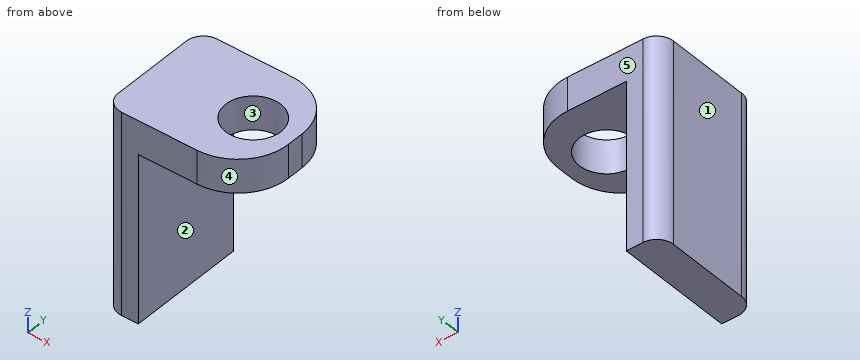
Autodesk Inventor part; units mm, degrees
ref_plane "YZ Plane" through (0, 0, 0) normal (1, 0, 0) x (0, 1, 0)
ref_plane "XZ Plane" through (0, 0, 0) normal (0, 1, 0) x (-1, 0, 0)
ref_plane "XY Plane" through (0, 0, 0) normal (0, 0, 1) x (1, 0, 0)
sketch "スケッチ1" plane through (0, 0, 0) normal (0, 0, 1) x (1, 0, 0)
  circle A0 centre (0, 0) radius 1.635
  line L0 (-6, -3.5) -> (2.5, -3.5)
  line L1 (2.5, -3.5) -> (2.5, 3.5)
  line L2 (2.5, 3.5) -> (-6, 3.5)
  line L3 (-6, 3.5) -> (-6, -3.5)
  line L4 (-6, -3.5) -> (2.5, 3.5) construction
  line L5 (2.5, -3.5) -> (-6, 3.5) construction
  line L6 (-6, 0) -> (2.5, 0) construction
  line L7 (-4, 3.5) -> (-4, -3.5)
  point P0 (-1.75, 0)
  dimension "d0" = 3.27
  dimension "d1" = 7
  dimension "d2" = 2.5
  dimension "d3" = 6
  dimension "d6" = 2
extrude "押し出し1" add sketch "スケッチ1" along normal blind 2
extrude "押し出し2" add sketch "スケッチ1" against normal blind 10 contours L3 L2 L7 L0
fillet "フィレット1" radius 3 2 edges at (2.5, 3.5, 1) (2.5, -3.5, 1)
fillet "フィレット2" radius 1 2 edges at (-6, -3.5, -4) (-6, 3.5, -4)
properties part number "guide_link"
Work out the finished part from the listing and answer in its coordinate system (mm). Face numbers are marked on the shaded views. A direction names the side the tool comes from. Give positions to 0.01 mm unless a question says otherwise; leave off trailing zeros. Order: outer loops, then holes, each group sorted by start corner. A loop starts at its lowest first (then second) coordinate and runs counter-clockwise, first axis right, second up. Notation, with made-up numbers: (34.25, -23) -> (55.25, -23) arc R20 cw to (55.25, 16) -> close; hole circle Ø10 at (55.25, -34.75). An arc over 180 degrees is marked (long way). Answer as a JSON object with one key per item and string values. Group by question number.
1. Section B-B on y = 0 is taken. Determine the outline of the cut face in (x, z) (3 decimals).
2. A flat-ended cylindrical pin translates along its axis: pin 1 Ø3 at (x, y) = (0.5, 1.5) entering from -Z. Find the tip coordinate at first contact, or state that the pin passes through.
3. Consider line 1 along Z through (x, y) = (-1.75, -1); line 2 along X through (y, z) = (-1.5, 0.5); line 3 along Y through (x, z) = (0, 1.3) (3 decimals). Determine where each line is inside the solid, lowest interval first. Write a range as [from, to].
4. A tool of negligible diameter and unlimited length cuts with its end or side. For the marked faces 1 and 2, from which of +Z, -Z, +X, -X, +Y, -Y can it reach the whole face along a straight path? Write none if from no direction.
5. Section C-C on x = 0 is taken. Determine the outline of the cut face in (y, z) (3 decimals), plus the area to 3 significant figures.
6. The mould has two halves that part along X. Classify the marked faces 3, 4 and 5: released by +X, released by -X, zero draft, split by the parting line, or undercut.
7. Section A-A on z = 0.5 is taken. Determine the outline of the cut face in (x, y) (3 decimals).
8. Section D-D on z = -9 is taken. Determine the outline of the cut face in (x, y), plus the area to 3 significant figures.
Result sheet:
{
 "1": {"outline": "(-6, -10) -> (-4, -10) -> (-4, 0) -> (-1.635, 0) -> (-1.635, 2) -> (-6, 2) -> close; (1.635, 0) -> (2.5, 0) -> (2.5, 2) -> (1.635, 2) -> close"},
 "2": {"pin 1": "stops at z = 0"},
 "3": {"line 1": "z = [0, 2]", "line 2": "x = [-6, -0.65], [0.65, 2.33]", "line 3": "y = [-3.458, -1.635], [1.635, 3.458]"},
 "4": {"face 1": "+Z, -Z, -X, +Y, -Y", "face 2": "-Z, +X, +Y, -Y"},
 "5": {"outline": "(-3.458, 0) -> (-1.635, 0) -> (-1.635, 2) -> (-3.458, 2) -> close; (1.635, 0) -> (3.458, 0) -> (3.458, 2) -> (1.635, 2) -> close", "area": "7.29 mm^2"},
 "6": {"face 3": "undercut", "face 4": "released by +X", "face 5": "zero draft"},
 "7": {"outline": "(-6, -2.5) arc R1 ccw to (-5, -3.5) -> (-0.5, -3.5) arc R3 ccw to (2.5, -0.5) -> (2.5, 0.5) arc R3 ccw to (-0.5, 3.5) -> (-5, 3.5) arc R1 ccw to (-6, 2.5) -> close; hole circle Ø3.27 at (0, 0)"},
 "8": {"outline": "(-6, -2.5) arc R1 ccw to (-5, -3.5) -> (-4, -3.5) -> (-4, 3.5) -> (-5, 3.5) arc R1 ccw to (-6, 2.5) -> close", "area": "13.6 mm^2"}
}
